```python
from build123d import *

# Parameters (mm, degrees)
SKETCH_1_W           = 80
SKETCH_1_H           = 100
EXTRUDE_1_DEPTH      = 100
SKETCH_2_W           = 80
SKETCH_2_H           = 85
CUT_EXTRUDE_1_DEPTH  = 90
CUT_EXTRUDE_5_DEPTH  = 138.477270849
SHELL_2_T            = -2
FILLET_1_R           = 3
FILLET_2_R           = 5
FILLET_3_R           = 3
SKETCH_6_W           = 3.8
SKETCH_6_H           = 2.5
CUT_EXTRUDE_6_DEPTH  = 85
SKETCH_8_W           = 5
SKETCH_8_H           = 5
CUT_EXTRUDE_7_DEPTH  = 100
SKETCH_11_W          = 2
SKETCH_11_H          = 1
CUT_EXTRUDE_8_DEPTH  = 119.74342103
SCALE_1_SCALE        = 5
SKETCH_12_W          = 400
SKETCH_12_H          = 300
SKETCH_12_W_2        = 185
SKETCH_12_H_2        = 29.670884313
CUT_EXTRUDE_11_DEPTH = 594.717104512
SKETCH_15_W          = 190
SKETCH_15_H          = 190
SKETCH_15_H_2        = 200
SKETCH_15_W_2        = 10
CUT_EXTRUDE_13_DEPTH = 575.45626481


with BuildPart() as part:
    # 스케치1 → 보스-돌출1 (new body)
    with BuildSketch(Plane.XY):
        Rectangle(SKETCH_1_W, SKETCH_1_H)
    extrude(amount=-EXTRUDE_1_DEPTH)

    # 스케치2 → 컷-돌출1 (cut)
    with BuildSketch(Plane(origin=(40, 0, 0), x_dir=(0, 0, -1), z_dir=(1, 0, 0))):
        with Locations((40, 7.5)):
            Rectangle(SKETCH_2_W, SKETCH_2_H)
    extrude(amount=-CUT_EXTRUDE_1_DEPTH, mode=Mode.SUBTRACT)

    # 스케치5 → 컷-돌출5 (cut, through all)
    with BuildSketch(Plane(origin=(40, 0, 0), x_dir=(0, 0, -1), z_dir=(1, 0, 0))):
        with BuildLine():
            add(Edge.make_bspline(
                [(0, -39.376697629), (18.60893103, -37.813832642), (60.522018707, -41.448787519), (82.629316251, -41.815039561), (94.476954899, -29.981594577), (72.35205171, -11.407179683), (96, 50)],
                knots=[0, 0, 0, 0, 0.361871867, 0.526261735, 0.755385015, 1, 1, 1, 1], degree=3))
            Line((96, 50), (80, 50))
            Line((80, 50), (80, -35))
            Line((80, -35), (0, -35))
            Line((0, -35), (0, -39.376697629))
        make_face()
    extrude(amount=-CUT_EXTRUDE_5_DEPTH, mode=Mode.SUBTRACT)

    # 쉘2
    shell_2_openings = [part.faces().sort_by_distance(p)[0] for p in [
        (0, 0, -100),
        (0, -50, -50),
    ]]
    offset(amount=SHELL_2_T, openings=shell_2_openings, kind=Kind.INTERSECTION)

    # 필렛1
    fillet_1_edges = [part.edges().sort_by_distance(p)[0] for p in [
        (0, 50, -96),
    ]]
    fillet(fillet_1_edges, radius=FILLET_1_R)

    # 필렛2
    fillet_2_edges = [part.edges().sort_by_distance(p)[0] for p in [
        (0, -39.376697629, 0),
    ]]
    fillet(fillet_2_edges, radius=FILLET_2_R)

    # 필렛3
    fillet_3_edges = [part.edges().sort_by_distance(p)[0] for p in [
        (40, -47.032911569, 0),
        (40, 49.469386486, -96.360930071),
        (-40, 49.469386486, -96.360930071),
        (40, -34.292790316, -87.583679146),
        (-40, -34.292790311, -87.583679133),
        (40, -40.61329303, -1.383366779),
        (-40, -47.032911569, 0),
        (-40, -40.61329303, -1.383366779),
        (-40, 50, -99.032247048),
        (40, 50, -99.032247048),
    ]]
    fillet(fillet_3_edges, radius=FILLET_3_R)

    # 스케치6 → 컷-돌출6 (cut)
    with BuildSketch(Plane(origin=(0, 0, -100), x_dir=(-1, 0, 0), z_dir=(0, 0, -1))):
        with Locations((-10, 10)):
            Rectangle(SKETCH_6_W, SKETCH_6_H)
        with Locations((10, 10)):
            Rectangle(SKETCH_6_W, SKETCH_6_H)
    extrude(amount=-CUT_EXTRUDE_6_DEPTH, mode=Mode.SUBTRACT)

    # 스케치8 → 컷-돌출7 (cut)
    with BuildSketch(Plane(origin=(0, 50, 0), x_dir=(1, 0, 0), z_dir=(0, 1, 0))):
        with Locations((-20, 69.358931696)):
            Rectangle(SKETCH_8_W, SKETCH_8_H)
        with Locations((20, 69.358931696)):
            Rectangle(SKETCH_8_W, SKETCH_8_H)
    extrude(amount=-CUT_EXTRUDE_7_DEPTH, mode=Mode.SUBTRACT)

    # 스케치11 → 컷-돌출8 (cut, through all)
    with BuildSketch(Plane(origin=(0, 0, -100), x_dir=(-1, 0, 0), z_dir=(0, 0, -1))):
        with Locations((-10, 3.626900341)):
            Rectangle(SKETCH_11_W, SKETCH_11_H)
        with Locations((10, 3.626900341)):
            Rectangle(SKETCH_11_W, SKETCH_11_H)
    extrude(amount=-CUT_EXTRUDE_8_DEPTH, mode=Mode.SUBTRACT)


with BuildPart() as part_1:
    # 축척1: scaled about (0, 0, 0)
    add(part.part.scale(SCALE_1_SCALE))

    # 스케치12 → 컷-돌출11 (cut, through all)
    with BuildSketch(Plane.XY):
        with Locations((0, 100)):
            Rectangle(SKETCH_12_W, SKETCH_12_H)
        Polygon((0, -50), (-200, -50), (-200, -250), (-185, -250), (-185, -220.329115687), (0, -220.329115687), align=None)
        with Locations((-92.5, -235.164557844)):
            Rectangle(SKETCH_12_W_2, SKETCH_12_H_2)
    extrude(amount=-CUT_EXTRUDE_11_DEPTH, mode=Mode.SUBTRACT)

    # 스케치15 → 컷-돌출13 (cut, through all)
    with BuildSketch(Plane.XZ.offset(250)):
        with Locations((95, -105)):
            Rectangle(SKETCH_15_W, SKETCH_15_H)
        with BuildLine():
            Line((190, -200), (200, -200))
            Line((200, -200), (200, -15))
            ThreePointArc((200, -15), (195.606601718, -4.393398282), (185, 0))
            Line((185, 0), (0, 0))
            Line((0, 0), (0, -10))
            Line((0, -10), (190, -10))
            Line((190, -10), (190, -200))
        make_face()
        with Locations((95, -400)):
            Rectangle(SKETCH_15_W, SKETCH_15_H_2)
        with Locations((195, -400)):
            Rectangle(SKETCH_15_W_2, SKETCH_15_H_2)
    extrude(amount=-CUT_EXTRUDE_13_DEPTH, mode=Mode.SUBTRACT)


solid = part_1.part
```
Can you work these out from the model? Positions are in its coordinate system, mm. Coordinates: 2 decimals unless noted, no trailing zeros. Order: outer loops, then holes, each group sorted by start corner. A loop starts at its lowest first (then second) coordinate and runs counter-clockwise, first axis right, second up. Notation, with made-up numbers: (51, 60.5) -> (79, 60.5) arc R24 ccw to (79, 89.5) -> close; hole circle Ø2 at (4.5, -10.75). An arc over 180 degrees is marked (long way). Write each question's results on one line, items separated by ' | '.
Item 1: I want a section at A-A, the plane y = -231. Write out the boundary of the cut face in (x, z).
Results are:
outline: (190, -300) -> (200, -300) -> (200, -200) -> (190, -200) -> close
Item 2: I'm going to push flat-ended pins straight in: pin 1 Ø5 at (y, z) = (-233.5, -236) entering from -X; pin 2 Ø10 at (x, z) = (107.5, -224) entering from +Y; pin 3 Ø5 at (y, z) = (-209.5, -279.5) entering from +X. Where does each tip first touch, or does it pass through?
Results are:
pin 1: x = 190 | pin 2: y = -199.86 | pin 3: x = 198.42
Item 3: If I drill on line 1 along X through (y, z) = (-235, -223); line 2 along X through (y, z) = (-213.5, -219.5); line 3 along Y through (x, z) = (149.5, -232), over which ranges is the centre line in solid material (lowest first)?
Results are:
line 1: 190 to 200 | line 2: 190 to 199.93 | line 3: -210.68 to -200.66
